from build123d import *

# Parameters (mm, degrees)
BOSS_EXTRUDE1_DEPTH = 60
CUT_EXTRUDE2_REACH  = 161.501
SKETCH2_R           = 1.425
CUT_EXTRUDE3_REACH  = 115.849
SKETCH10_R          = 5
SKETCH10_R_2        = 4
SKETCH10_R_3        = 2
BOSS_EXTRUDE2_DEPTH = 11
BOSS_EXTRUDE3_DEPTH = 11
FILLET2_R           = 10
FILLET3_R           = 10
FILLET4_R           = 5
FILLET5_R           = 5
FILLET6_R           = 2.5
FILLET7_R           = 2.5
FILLET8_START       = -61
FILLET8_DEPTH       = 62
FILLET9_R           = 6


with BuildPart() as part:
    # Sketch1 → Boss-Extrude1 (new body)
    with BuildSketch(Plane(origin=(0, 0, 0), x_dir=(0, 0, -1), z_dir=(1, 0, 0))):
        Polygon((-20.469264339, 61.494964584), (-20.469264339, 66.494964584), (39.530735661, 66.494964584), (39.530735661, -75.905035416), (34.530735661, -75.905035416), (34.530735661, 61.494964584), align=None)
    extrude(amount=-BOSS_EXTRUDE1_DEPTH)

    # Sketch2 → Cut-Extrude2 (cut, up to next)
    with BuildSketch(Plane(origin=(0, 66.494964584, 0), x_dir=(1, 0, 0), z_dir=(0, 1, 0)), mode=Mode.PRIVATE) as cut_extrude2_sk1:
        with Locations(Location((-35.5, 10.030735661, 0), (0, 0, 270))):
            Circle(SKETCH2_R)
    cut_extrude2_tool1 = extrude(cut_extrude2_sk1.sketch, amount=-CUT_EXTRUDE2_REACH, mode=Mode.PRIVATE) & part.part
    # Sketch2 → Cut-Extrude2 (cut, up to next)
    with BuildSketch(Plane(origin=(0, 66.494964584, 0), x_dir=(1, 0, 0), z_dir=(0, 1, 0)), mode=Mode.PRIVATE) as cut_extrude2_sk2:
        with Locations(Location((-24.5, 10.030735661, 0), (0, 0, 270))):
            Circle(SKETCH2_R)
    cut_extrude2_tool2 = extrude(cut_extrude2_sk2.sketch, amount=-CUT_EXTRUDE2_REACH, mode=Mode.PRIVATE) & part.part
    # Sketch2 → Cut-Extrude2 (cut, up to next)
    with BuildSketch(Plane(origin=(0, 66.494964584, 0), x_dir=(1, 0, 0), z_dir=(0, 1, 0)), mode=Mode.PRIVATE) as cut_extrude2_sk3:
        with Locations(Location((-24.5, -0.969264339, 0), (0, 0, 270))):
            Circle(SKETCH2_R)
    cut_extrude2_tool3 = extrude(cut_extrude2_sk3.sketch, amount=-CUT_EXTRUDE2_REACH, mode=Mode.PRIVATE) & part.part
    # Sketch2 → Cut-Extrude2 (cut, up to next)
    with BuildSketch(Plane(origin=(0, 66.494964584, 0), x_dir=(1, 0, 0), z_dir=(0, 1, 0)), mode=Mode.PRIVATE) as cut_extrude2_sk4:
        with Locations(Location((-35.5, -0.969264339, 0), (0, 0, 270))):
            Circle(SKETCH2_R)
    cut_extrude2_tool4 = extrude(cut_extrude2_sk4.sketch, amount=-CUT_EXTRUDE2_REACH, mode=Mode.PRIVATE) & part.part
    add(cut_extrude2_tool1.solids().sort_by_distance((-35.5, 66.494965, -10.030736))[0], mode=Mode.SUBTRACT)
    add(cut_extrude2_tool2.solids().sort_by_distance((-24.5, 66.494965, -10.030736))[0], mode=Mode.SUBTRACT)
    add(cut_extrude2_tool3.solids().sort_by_distance((-24.5, 66.494965, 0.969264))[0], mode=Mode.SUBTRACT)
    add(cut_extrude2_tool4.solids().sort_by_distance((-35.5, 66.494965, 0.969264))[0], mode=Mode.SUBTRACT)

    # Sketch10 → Cut-Extrude3 (cut, up to next)
    with BuildSketch(Plane(origin=(0, 0, -39.530735661), x_dir=(-1, 0, 0), z_dir=(0, 0, -1)), mode=Mode.PRIVATE) as cut_extrude3_sk1:
        with Locations(Location((30, 33.994964584, 0), (0, 0, 90))):
            Circle(SKETCH10_R)
    cut_extrude3_tool1 = extrude(cut_extrude3_sk1.sketch, amount=-CUT_EXTRUDE3_REACH, mode=Mode.PRIVATE) & part.part
    # Sketch10 → Cut-Extrude3 (cut, up to next)
    with BuildSketch(Plane(origin=(0, 0, -39.530735661), x_dir=(-1, 0, 0), z_dir=(0, 0, -1)), mode=Mode.PRIVATE) as cut_extrude3_sk2:
        with Locations(Location((30, -38.005035416, 0), (0, 0, 90))):
            Circle(SKETCH10_R_2)
    cut_extrude3_tool2 = extrude(cut_extrude3_sk2.sketch, amount=-CUT_EXTRUDE3_REACH, mode=Mode.PRIVATE) & part.part
    # Sketch10 → Cut-Extrude3 (cut, up to next)
    with BuildSketch(Plane(origin=(0, 0, -39.530735661), x_dir=(-1, 0, 0), z_dir=(0, 0, -1)), mode=Mode.PRIVATE) as cut_extrude3_sk3:
        with Locations(Location((14.5, 49.494964584, 0), (0, 0, 90))):
            Circle(SKETCH10_R_3)
    cut_extrude3_tool3 = extrude(cut_extrude3_sk3.sketch, amount=-CUT_EXTRUDE3_REACH, mode=Mode.PRIVATE) & part.part
    # Sketch10 → Cut-Extrude3 (cut, up to next)
    with BuildSketch(Plane(origin=(0, 0, -39.530735661), x_dir=(-1, 0, 0), z_dir=(0, 0, -1)), mode=Mode.PRIVATE) as cut_extrude3_sk4:
        with Locations(Location((14.5, 18.494964584, 0), (0, 0, 90))):
            Circle(SKETCH10_R_3)
    cut_extrude3_tool4 = extrude(cut_extrude3_sk4.sketch, amount=-CUT_EXTRUDE3_REACH, mode=Mode.PRIVATE) & part.part
    # Sketch10 → Cut-Extrude3 (cut, up to next)
    with BuildSketch(Plane(origin=(0, 0, -39.530735661), x_dir=(-1, 0, 0), z_dir=(0, 0, -1)), mode=Mode.PRIVATE) as cut_extrude3_sk5:
        with Locations(Location((45.5, 18.494964584, 0), (0, 0, 90))):
            Circle(SKETCH10_R_3)
    cut_extrude3_tool5 = extrude(cut_extrude3_sk5.sketch, amount=-CUT_EXTRUDE3_REACH, mode=Mode.PRIVATE) & part.part
    # Sketch10 → Cut-Extrude3 (cut, up to next)
    with BuildSketch(Plane(origin=(0, 0, -39.530735661), x_dir=(-1, 0, 0), z_dir=(0, 0, -1)), mode=Mode.PRIVATE) as cut_extrude3_sk6:
        with Locations(Location((45.5, 49.494964584, 0), (0, 0, 90))):
            Circle(SKETCH10_R_3)
    cut_extrude3_tool6 = extrude(cut_extrude3_sk6.sketch, amount=-CUT_EXTRUDE3_REACH, mode=Mode.PRIVATE) & part.part
    # Sketch10 → Cut-Extrude3 (cut, up to next)
    with BuildSketch(Plane(origin=(0, 0, -39.530735661), x_dir=(-1, 0, 0), z_dir=(0, 0, -1)), mode=Mode.PRIVATE) as cut_extrude3_sk7:
        with Locations(Location((5, 1.994964584, 0), (0, 0, 90))):
            Circle(SKETCH10_R_3)
    cut_extrude3_tool7 = extrude(cut_extrude3_sk7.sketch, amount=-CUT_EXTRUDE3_REACH, mode=Mode.PRIVATE) & part.part
    # Sketch10 → Cut-Extrude3 (cut, up to next)
    with BuildSketch(Plane(origin=(0, 0, -39.530735661), x_dir=(-1, 0, 0), z_dir=(0, 0, -1)), mode=Mode.PRIVATE) as cut_extrude3_sk8:
        with Locations(Location((55, 1.994964584, 0), (0, 0, 90))):
            Circle(SKETCH10_R_3)
    cut_extrude3_tool8 = extrude(cut_extrude3_sk8.sketch, amount=-CUT_EXTRUDE3_REACH, mode=Mode.PRIVATE) & part.part
    # Sketch10 → Cut-Extrude3 (cut, up to next)
    with BuildSketch(Plane(origin=(0, 0, -39.530735661), x_dir=(-1, 0, 0), z_dir=(0, 0, -1)), mode=Mode.PRIVATE) as cut_extrude3_sk9:
        with Locations(Location((30, -70.905035416, 0), (0, 0, 90))):
            Circle(SKETCH10_R_3)
    cut_extrude3_tool9 = extrude(cut_extrude3_sk9.sketch, amount=-CUT_EXTRUDE3_REACH, mode=Mode.PRIVATE) & part.part
    add(cut_extrude3_tool1.solids().sort_by_distance((-30, 33.994965, -39.530736))[0], mode=Mode.SUBTRACT)
    add(cut_extrude3_tool2.solids().sort_by_distance((-30, -38.005035, -39.530736))[0], mode=Mode.SUBTRACT)
    add(cut_extrude3_tool3.solids().sort_by_distance((-14.5, 49.494965, -39.530736))[0], mode=Mode.SUBTRACT)
    add(cut_extrude3_tool4.solids().sort_by_distance((-14.5, 18.494965, -39.530736))[0], mode=Mode.SUBTRACT)
    add(cut_extrude3_tool5.solids().sort_by_distance((-45.5, 18.494965, -39.530736))[0], mode=Mode.SUBTRACT)
    add(cut_extrude3_tool6.solids().sort_by_distance((-45.5, 49.494965, -39.530736))[0], mode=Mode.SUBTRACT)
    add(cut_extrude3_tool7.solids().sort_by_distance((-5, 1.994965, -39.530736))[0], mode=Mode.SUBTRACT)
    add(cut_extrude3_tool8.solids().sort_by_distance((-55, 1.994965, -39.530736))[0], mode=Mode.SUBTRACT)
    add(cut_extrude3_tool9.solids().sort_by_distance((-30, -70.905035, -39.530736))[0], mode=Mode.SUBTRACT)

    # Sketch11 → Boss-Extrude2 (add)
    with BuildSketch(Plane(origin=(0, 0, 0), x_dir=(0, 0, -1), z_dir=(1, 0, 0))):
        Polygon((-15.469264339, 61.494964584), (34.530735661, 16.494964584), (34.530735661, 11.494964584), (-20.469264339, 61.494964584), align=None)
    extrude(amount=-BOSS_EXTRUDE2_DEPTH)

    # Sketch13 → Boss-Extrude3 (add)
    with BuildSketch(Plane.ZY.offset(60)):
        Polygon((-34.530735661, 11.494964584), (-34.530735661, 16.494964584), (15.469264339, 61.494964584), (20.469264339, 61.494964584), align=None)
    extrude(amount=-BOSS_EXTRUDE3_DEPTH)

    # Fillet2
    fillet2_edges = [part.edges().sort_by_distance(p)[0] for p in [
        (-54.5, 11.494964584, -34.530735661),
    ]]
    fillet(fillet2_edges, radius=FILLET2_R)

    # Fillet3
    fillet3_edges = [part.edges().sort_by_distance(p)[0] for p in [
        (-5.5, 11.494964584, -34.530735661),
    ]]
    fillet(fillet3_edges, radius=FILLET3_R)

    # Fillet4
    fillet4_edges = [part.edges().sort_by_distance(p)[0] for p in [
        (-5.5, 16.494964584, -34.530735661),
    ]]
    fillet(fillet4_edges, radius=FILLET4_R)

    # Fillet5
    fillet5_edges = [part.edges().sort_by_distance(p)[0] for p in [
        (-54.5, 16.494964584, -34.530735661),
    ]]
    fillet(fillet5_edges, radius=FILLET5_R)

    # Fillet6
    fillet6_edges = [part.edges().sort_by_distance(p)[0] for p in [
        (-54.5, 61.494964584, 15.469264339),
    ]]
    fillet(fillet6_edges, radius=FILLET6_R)

    # Fillet7
    fillet7_edges = [part.edges().sort_by_distance(p)[0] for p in [
        (-5.5, 61.494964584, 15.469264339),
    ]]
    fillet(fillet7_edges, radius=FILLET7_R)

    # Fillet8: read off the stored shape, not the designer's step
    # Fillet8 outline → Fillet8 (cut)
    with BuildSketch(Plane.YZ.offset(FILLET8_START)):
        with BuildLine():
            Line((61.494964584, 20.469264339), (60.751039115, 19.650946324))
            ThreePointArc((60.751039115, 19.650946324), (61.589505337, 20.255550078), (62.600889299, 20.469264339))
            Line((62.600889299, 20.469264339), (61.494964584, 20.469264339))
        make_face()
    extrude(amount=FILLET8_DEPTH, mode=Mode.SUBTRACT)

    # Fillet9
    fillet9_edges = [part.edges().sort_by_distance(p)[0] for p in [
        (-30, 61.494964584, -34.530735661),
    ]]
    fillet(fillet9_edges, radius=FILLET9_R)


solid = part.part
Here's how the part is built. I have some questions about the finished solid (model axes, mm). A direction names the side the tool comes from. Coordinates: 2 decimals unless noted, no trailing zeros. Order: outer loops, then holes, each group sorted by start corner. A loop starts at its lowest first (then second) coordinate and runs counter-clockwise, first axis right, second up. Notation, with made-up numbers: (23.25, 9.25) -> (61.25, 9.25) arc R29 cw to (61.25, 31.25) -> close; hole circle Ø1 at (54.5, 39). An arc over 180 degrees is marked (long way). Answer in a Markdown table with one row per item.
(1) Will these pins go through, and if not, where does the flat tip stop? pin 1 Ø24.5 at (x, z) = (-39.5, -12.5) entering from -Y; pin 2 Ø3.5 at (x, z) = (-24.5, -10.03) entering from +Y; pin 3 Ø6.5 at (x, y) = (-45.5, 18.49) entering from +Z.
Answer key:
| item | result |
|---|---|
| pin 1 | y = 24.49 |
| pin 2 | y = 66.49 |
| pin 3 | z = -34.53 |
(2) On a 3-axis mill with a long thin cutter (end or side, diameter ignored), from which of +Z, -Z, +X, -X, +Y, -Y can I reach the whole of each face in a straight line? I mean faces 3 (the face through (-34.087, 64.03, 0.784)), 4 (the face through (-54.423, 59.851, 11.303)), 5 (the face through (-49, 36, -11)). Say none if no direction works.
Answer key:
| item | result |
|---|---|
| face 3 | +Y, -Y |
| face 4 | +X, -X |
| face 5 | +Z, -Y |
(3) I want a section at C-C on z = -19. List the corners of the cut face in (x, y) for me.
Answer key:
| item | result |
|---|---|
| outline | (-60, 25.61) -> (-49, 25.61) -> (-49, 30.47) -> (-60, 30.47) -> close; (-60, 61.49) -> (0, 61.49) -> (0, 66.49) -> (-60, 66.49) -> close; (-11, 25.61) -> (0, 25.61) -> (0, 30.47) -> (-11, 30.47) -> close |
(4) I want a section at D-D on x = -45.5. List the corners of the cut face in (y, z) for me.
Answer key:
| item | result |
|---|---|
| outline | (-75.91, -39.53) -> (16.49, -39.53) -> (16.49, -34.53) -> (-75.91, -34.53) -> close; (20.49, -39.53) -> (47.49, -39.53) -> (47.49, -34.53) -> (20.49, -34.53) -> close; (51.49, -39.53) -> (66.49, -39.53) -> (66.49, 20.47) -> (62.6, 20.47) arc R2.5 ccw to (61.49, 20.21) -> (61.49, -28.53) arc R6 cw to (55.49, -34.53) -> (51.49, -34.53) -> close |
(5) Thinking about a two-plate mould opening in X: for faces 1 (the face through (-47.452, 18.061, -37.066)), 2 (the face through (-30.42, 59.78, -32.73)), which applies, +X half, -X half, draft (parallel to the pull), parting line (faces both ways), or undercut?
Answer key:
| item | result |
|---|---|
| face 1 | undercut |
| face 2 | draft |
(6) Please list where these lines run through material, in increasing order: probe 1 along Y at (x, z) = (-14, -37); probe 2 along Z at (x, y) = (-10.5, 10); probe 3 along Y at (x, z) = (-15.5, -7).
Answer key:
| item | result |
|---|---|
| probe 1 | -75.91 to 16.56, 20.43 to 47.56, 51.43 to 66.49 |
| probe 2 | -39.53 to -34.09 |
| probe 3 | 61.49 to 66.49 |
(7) I want a section at A-A on x = -30. List the corners of the cut face in (y, z) for me.
Answer key:
| item | result |
|---|---|
| outline | (-75.91, -39.53) -> (-72.91, -39.53) -> (-72.91, -34.53) -> (-75.91, -34.53) -> close; (-68.91, -39.53) -> (-42.01, -39.53) -> (-42.01, -34.53) -> (-68.91, -34.53) -> close; (-34.01, -39.53) -> (28.99, -39.53) -> (28.99, -34.53) -> (-34.01, -34.53) -> close; (38.99, -39.53) -> (66.49, -39.53) -> (66.49, 20.47) -> (62.6, 20.47) arc R2.5 ccw to (61.49, 20.21) -> (61.49, -28.53) arc R6 cw to (55.49, -34.53) -> (38.99, -34.53) -> close |
(8) I want a section at B-B on x = -55. List the corners of the cut face in (y, z) for me, then the cut area to 3 significant figures.
Answer key:
| item | result |
|---|---|
| outline | (-75.91, -39.53) -> (-0.01, -39.53) -> (-0.01, -34.53) -> (-75.91, -34.53) -> close; (3.99, -39.53) -> (66.49, -39.53) -> (66.49, 20.47) -> (62.6, 20.47) arc R2.5 ccw to (60.75, 19.65) -> (14.47, -31.26) arc R10 cw to (7.07, -34.53) -> (3.99, -34.53) -> close; hole (24.01, -26.19) arc R5 ccw to (27.72, -34.53) -> (55.49, -34.53) arc R6 ccw to (61.49, -28.53) -> (61.49, 8.95) arc R2.5 ccw to (57.14, 10.63) -> close |
| area | 1,260 mm^2 |
